Check sheet for the modelled part. Datum: model origin and axes. Units: mm. A direction names the side the tool comes from. Round coordinates to 2 decimals unless told otherwise and drop trailing zeros. Loops run counter-clockwise (first coordinate to the right, second up) from the corner with the lowest first, then second, coordinate; pieces in that order, holes last. Notation, with made-up numbers: (65, -19.75) - (108, -19.75) arc R8 ccw to (108, -7.75) - close; hole circle Ø2 at (78, 1.5). An arc over 180 degrees is marked (long way). Put each result on its own line as item: value. Start each with the question number.
Item 1: Section check D-D, the plane z = 4.25. Record the cut outline in (x, y).
Item 2: Material ranges on line 1 along Y through (x, z) = (35, -1.3); line 2 along X through (y, z) = (-20, -2); line 3 along X through (y, z) = (-5.5, 9.75), recorded low to high.
Item 3: Tool access check on faces 5 (the flat face through (-10, -1, 8)), 6 (the flat face through (2, -20, 12)), 7 (the flat face through (-28, -1, 0)). Record the directions out of +Z, -Z, +X, -X, +Y, -Y that give a thin tool (end or side, any length) a straight path to the whole face; none if there is none.
Item 4: Section check C-C, the plane x = -11. Record the cut outline in (y, z).
Item 5: Gauge pin test, flat ends, axial feed: pin 1 Ø10 at (y, z) = (-5.5, 12) entering from +X; pin 2 Ø4 at (x, y) = (30.5, 23) entering from +Z; pin 3 Ø10 at (y, z) = (-3.5, 8) entering from -X. Record the tip position at first contact, or that the pin passes through.
Item 6: Draft check along X on faces 1 (the flat face through (2, 20, 12)), 2 (the flat face through (-15, -1, 8)), 3 (the flat face through (0, -1, 8)), 4 (the cylindrical face through (32, 20, -2)). Enter one of: pulls with the +X half, pulls with the -X half, needs draft (parallel to the pull), parting line crosses it, or undercut.
Item 7: Section check A-A, the plane y = -15. Record the cut outline in (x, z), and give its area (3 significant figures).
Item 8: Section check B-B, the plane x = 35. Record the cut outline in (y, z), and give its area (3 significant figures).
from build123d import *

# Parameters (mm, degrees)
F0_W      = 5
F0_H      = 20
F1_DEPTH  = 40
F2_R      = 2
F3_R      = 2
F4_W      = 40
F4_H      = 5
F5_DEPTH  = 25
F6_W      = 10
F6_H      = 80
F7_DEPTH  = 3
F8_R      = 3
F9_DEPTH  = 3
F12_R     = 10
F13_DEPTH = 25


with BuildPart() as f1:
    # F0 (on Front) → F1 (new body, symmetric)
    with BuildSketch(Plane.XZ):
        with Locations((-12.5, 10)):
            Rectangle(F0_W, F0_H)
        Polygon((0, 0), (-10, 0), (-15, 0), (-40, 0), (-40, -5), (0, -5), align=None)
        with Locations((2.5, 10)):
            Rectangle(F0_W, F0_H)
        Polygon((5, 0), (0, 0), (0, -5), (30, -5), (30, 0), align=None)
    extrude(amount=F1_DEPTH, both=True)

    # F2
    f2_edges = [f1.edges().sort_by_distance(p)[0] for p in [
        (5, 0, 0),
        (-15, 0, 0),
    ]]
    fillet(f2_edges, radius=F2_R)

    # F3
    f3_edges = [f1.edges().sort_by_distance(p)[0] for p in [
        (-15, 0, 20),
        (5, 0, 20),
    ]]
    fillet(f3_edges, radius=F3_R)

    # F4 (on face) → F5 (cut)
    with BuildSketch(Plane(origin=(-15, 0, 0), x_dir=(0, -1, 0), z_dir=(-1, 0, 0))):
        with Locations((0, 12.5)):
            Rectangle(F4_W, F4_H)
    extrude(amount=-F5_DEPTH, mode=Mode.SUBTRACT)

    # F6 (on face) → F7 (join)
    with BuildSketch(Plane.XY):
        with Locations((35, 0)):
            Rectangle(F6_W, F6_H)
    extrude(amount=-F7_DEPTH)


with BuildPart() as f9:
    # F8 (on face) → F9 (new body)
    with BuildSketch(Plane(origin=(0, 0, -3), x_dir=(1, 0, 0), z_dir=(0, 0, -1))):
        with Locations((35, 20)):
            Circle(F8_R)
    extrude(amount=-F9_DEPTH)


with BuildPart() as f10_1:
    # F10: instance of F9
    add(f9.part.mirror(Plane.XZ))


with BuildPart() as f1_1:
    add(f1.part)

    # F11: cut F10_1, F9
    add(f10_1.part, mode=Mode.SUBTRACT)
    add(f9.part, mode=Mode.SUBTRACT)

    # F12 (on face) → F13 (cut)
    with BuildSketch(Plane(origin=(-15, 0, 0), x_dir=(0, -1, 0), z_dir=(-1, 0, 0))):
        with Locations((0, 28)):
            Circle(F12_R)
    extrude(amount=-F13_DEPTH, mode=Mode.SUBTRACT)


solid = f1_1.part
Check result:
1. outline: (-15, -40) - (-10, -40) - (-10, 40) - (-15, 40) - close; (0, -40) - (5, -40) - (5, 40) - (0, 40) - close
2. line 1: -40 to -23, -17 to 17, 23 to 40
2. line 2: -40 to 32, 38 to 40
2. line 3: -15 to -10, 0 to 5
3. face 5: +Z, +Y, -Y
3. face 6: +X, -X
3. face 7: +Z, -X, +Y, -Y
4. outline: (-40, -5) - (40, -5) - (40, 20) - (6, 20) arc R10 cw to (-6, 20) - (-40, 20) - close; hole (-20, 10) - (20, 10) - (20, 15) - (-20, 15) - close
5. pin 1: x = 5
5. pin 2: z = 0
5. pin 3: x = -15
6. face 1: needs draft
6. face 2: pulls with the -X half
6. face 3: undercut
6. face 4: undercut
7. outline: (-40, -5) - (30, -5) - (30, -3) - (40, -3) - (40, 0) - (7, 0) arc R2 cw to (5, 2) - (5, 10) - (0, 10) - (0, 0) - (-10, 0) - (-10, 10) - (-15, 10) - (-15, 2) arc R2 cw to (-17, 0) - (-40, 0) - close; (-15, 15) - (-10, 15) - (-10, 20) - (-13, 20) arc R2 ccw to (-15, 18) - close; (0, 15) - (5, 15) - (5, 18) arc R2 ccw to (3, 20) - (0, 20) - close
7. area: 530 mm²
8. outline: (-40, -3) - (-23, -3) - (-23, 0) - (-40, 0) - close; (-17, -3) - (17, -3) - (17, 0) - (-17, 0) - close; (23, -3) - (40, -3) - (40, 0) - (23, 0) - close
8. area: 204 mm²
